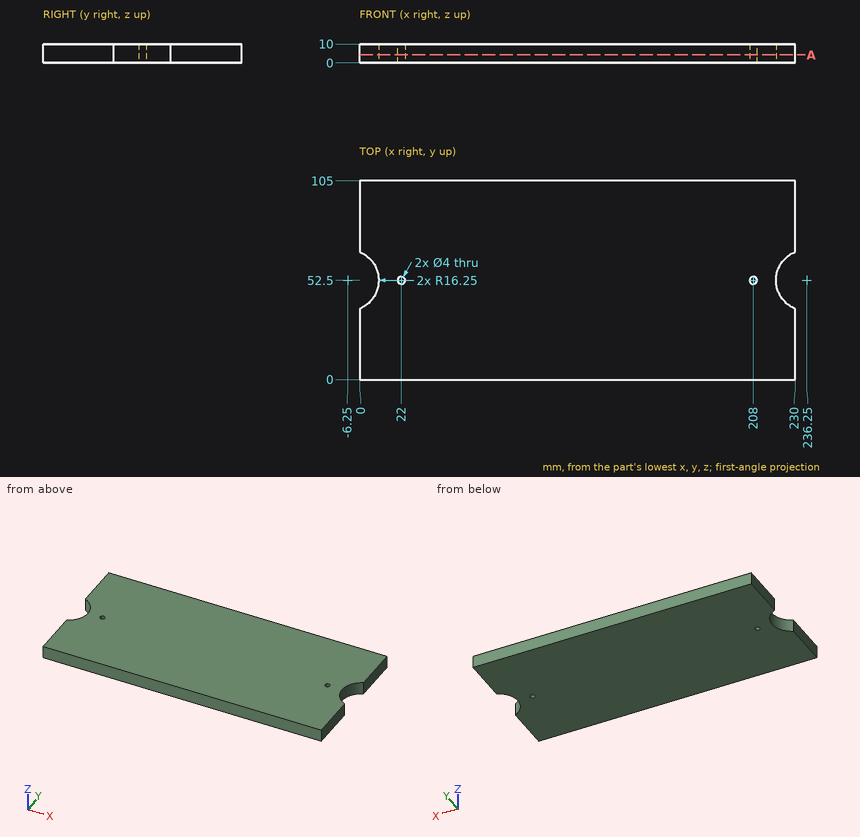
Drawing for the job (mm, zero at the part's lowest x, y, z). Give positions to 0.01 mm unless a question says otherwise; leave off trailing zeros. Loops run counter-clockwise (first coordinate to the right, second up) from the corner with the lowest first, then second, coordinate; pieces in that order, holes last.
Item 1: Slice it at A-A (z = 4.25). Write the cut outline in (x, y), plus the area to 3 significant figures.
Check values:
outline: (0, 0) - (230, 0) - (230, 37.5) arc R16.25 cw to (230, 67.5) - (230, 105) - (0, 105) - (0, 67.5) arc R16.25 cw to (0, 37.5) - close; hole circle Ø4 at (22, 52.5); hole circle Ø4 at (208, 52.5)
area: 23,700 mm2
Item 2: Drop a flat-ended pin along its axis: P1, Ø3.5, axis at x = 22, y = 52.5, coming from the -Z side. Give the stop position or say it passes through.
Check values:
P1: passes through
Item 3: Drill centre lines: line 1 along Y through (x, z) = (208, 2.75); line 2 along Y through (x, z) = (20.5, 1); line 3 along X through (y, z) = (42.5, 3.5). Where is each one in solid material? Low to high.
Check values:
line 1: y = 0 to 50.5, 54.5 to 105
line 2: y = 0 to 51.18, 53.82 to 105
line 3: x = 6.56 to 223.44
